Design review of the part built by this model. Coordinates are the model's own, in mm. A direction names the side the tool comes from. Give positions to 0.01 mm unless a question says otherwise; leave off trailing zeros. Order: outer loops, then holes, each group sorted by start corner. A loop starts at its lowest first (then second) coordinate and runs counter-clockwise, first axis right, second up. Notation, with made-up numbers: M 4,73 L 24,73 A17 ccw 24,101 Z; hole C 59.5,-35 d2. An arc over 180 degrees is marked long. Answer as a JSON object with one key per item and string values.
from build123d import *

# Parameters (mm, degrees)
F0_W     = 63.5
F0_H     = 111.76
F1_DEPTH = 63.5
F3_T     = -2.54
F2_W     = 58.42
F2_H     = 48.26
F4_DEPTH = 25.4
F5_R     = 5.08
F6_DEPTH = 254


with BuildPart() as f1:
    # F0 (on Front) → F1 (new body)
    with BuildSketch(Plane.XZ):
        with Locations((0, -24.453788)):
            Rectangle(F0_W, F0_H)
    extrude(amount=-F1_DEPTH)

    # F3
    f3_openings = [f1.faces().sort_by_distance(p)[0] for p in [
        (0, 31.75, 31.426212),
    ]]
    offset(amount=F3_T, openings=f3_openings)

    # F2 (on face) → F4 (cut)
    with BuildSketch(Plane.XZ):
        with Locations((0, 7.296212)):
            Rectangle(F2_W, F2_H)
    extrude(amount=-F4_DEPTH, mode=Mode.SUBTRACT)

    # F5 (on face) → F6 (cut)
    with BuildSketch(Plane.XZ):
        with Locations((-15.24, -34.613788)):
            Circle(F5_R)
        with Locations((15.24, -34.613788)):
            Circle(F5_R)
    extrude(amount=-F6_DEPTH, mode=Mode.SUBTRACT)


solid = f1.part
(1) Tool access review of faces 5 (the flat face through (0, 1, -16.834)), 6 (the cylindrical face through (14.139, 62.212, -39.573)), 7 (the flat face through (0, 60.96, -22)): name each direction out of +Z, -Z, +X, -X, +Y, -Y from which nothing blocks a thin tool from reaching the whole face with its end or side.
Checked values:
{"face 5": "+Z, -Y", "face 6": "+Y, -Y", "face 7": "+Z"}
(2) We need section D-D (x = 24). Write out the cut boundary in (y, z).
Checked values:
{"outline": "M 0,-80.33 L 63.5,-80.33 L 63.5,31.43 L 60.96,31.43 L 60.96,-77.79 L 2.54,-77.79 L 2.54,-16.83 L 0,-16.83 Z"}
(3) Draft analysis for pull direction Z (two halves, no side actions). For faces 1 (the flat face through (0, 0, -49)), 2 (the cylindrical face through (-12.896, 62.212, -39.121)), 3 (the flat face through (0, 31, -77.794)), 4 (the flat face through (0, 31, -80.334)), state which applies: +Z half, -Z half, draft (parallel to the pull), parting line (faces both ways), or undercut.
Checked values:
{"face 1": "draft", "face 2": "undercut", "face 3": "+Z half", "face 4": "-Z half"}
(4) We need section B-B (z = -56.5). Write out the cut boundary in (x, y).
Checked values:
{"outline": "M -31.75,0 L 31.75,0 L 31.75,63.5 L -31.75,63.5 Z; hole M -29.21,2.54 L 29.21,2.54 L 29.21,60.96 L -29.21,60.96 Z"}
(5) We need section A-A (x = -15.24). Write out the cut boundary in (y, z), plus the area to 3 significant figures.
Checked values:
{"outline": "M 0,-80.33 L 63.5,-80.33 L 63.5,-39.69 L 60.96,-39.69 L 60.96,-77.79 L 2.54,-77.79 L 2.54,-39.69 L 0,-39.69 Z; M 0,-29.53 L 2.54,-29.53 L 2.54,-16.83 L 0,-16.83 Z; M 60.96,-29.53 L 63.5,-29.53 L 63.5,31.43 L 60.96,31.43 Z", "area": "542 mm^2"}
(6) Insertion check: pin 1 (2 mm diameter, centred on x = -19.5, y = 15, fed in from +Z); pin 2 (4 mm diameter, centred on x = -14, z = 10.5, fed in from -Y); pin 3 (8 mm diameter, centred on x = -15.24, z = -34.61, fed in from +Y); pin 4 (3 mm diameter, centred on x = 11.5, y = 1.5, fed in from +Z). Each pin has a flat end and moves straight along its axis. Give the tip position at first contact, or say it passes through.
Checked values:
{"pin 1": "stops at z = -77.79", "pin 2": "stops at y = 60.96", "pin 3": "passes through", "pin 4": "stops at z = -16.83"}
(7) We need section C-C (y = 36). Write out the cut boundary in (x, z).
Checked values:
{"outline": "M -31.75,-80.33 L 31.75,-80.33 L 31.75,31.43 L 29.21,31.43 L 29.21,-77.79 L -29.21,-77.79 L -29.21,31.43 L -31.75,31.43 Z"}
(8) To check wall thickness, follow L1, parallel to X at y = 8.5, z = 12.5; L2, parallel to Z at x = 15.24, y = 61.65; L3, parallel to Z at x = 15.24, y = 0.85. State the ranges of each line that lie inside material, in increasing order. Write a range as from..to.
Checked values:
{"L1": "x = -31.75..-29.21, 29.21..31.75", "L2": "z = -80.33..-39.69, -29.53..31.43", "L3": "z = -80.33..-39.69, -29.53..-16.83"}
